The listing builds one solid part. Answer for the finished solid, in the listing's coordinates (mm). A direction names the side the tool comes from. Coordinates: 2 decimals unless noted, no trailing zeros. Write each loop counter-clockwise with the first axis right and the second up, starting at its lowest first coordinate (ties: lowest second). Pieces come first, ordered by that corner, then holes. Notation, with made-up numbers: M 28,7.5 L 32,7.5 A19 ccw 32,23.5 Z; hole C 88,-32.75 d6. An arc over 180 degrees is marked long. Answer as CSV lines item,"result".
```python
from build123d import *

# Parameters (mm, degrees)
F0_W     = 306.0534086764
F0_H     = 101.6
F0_W_2   = 101.6
F0_H_2   = 152.4
F0_W_3   = 100.3465913236
F1_DEPTH = 25.4


with BuildPart() as f1:
    # F0 (on Top) → F1 (new body)
    with BuildSketch(Plane.XY):
        with Locations((220.9462343127, 820.6196134418)):
            Rectangle(F0_W, F0_H)
        with Locations((220.9462343127, 566.6196134418)):
            Rectangle(F0_W, F0_H)
        with Locations((220.9462343127, 312.6196134418)):
            Rectangle(F0_W, F0_H)
        with Locations((220.9462343127, 58.6196134418)):
            Rectangle(F0_W, F0_H)
        with Locations((424.7729386508, 58.6196134418)):
            Rectangle(F0_W_2, F0_H)
        with Locations((424.7729386508, 185.6196134418)):
            Rectangle(F0_W_2, F0_H_2)
        with Locations((424.7729386508, 312.6196134418)):
            Rectangle(F0_W_2, F0_H)
        with Locations((424.7729386508, 439.6196134418)):
            Rectangle(F0_W_2, F0_H_2)
        with Locations((424.7729386508, 566.6196134418)):
            Rectangle(F0_W_2, F0_H)
        with Locations((424.7729386508, 693.6196134418)):
            Rectangle(F0_W_2, F0_H_2)
        with Locations((424.7729386508, 820.6196134418)):
            Rectangle(F0_W_2, F0_H)
        with Locations((17.7462343127, 820.6196134418)):
            Rectangle(F0_W_3, F0_H)
        with Locations((17.7462343127, 693.6196134418)):
            Rectangle(F0_W_3, F0_H_2)
        with Locations((17.7462343127, 566.6196134418)):
            Rectangle(F0_W_3, F0_H)
        with Locations((17.7462343127, 439.6196134418)):
            Rectangle(F0_W_3, F0_H_2)
        with Locations((17.7462343127, 312.6196134418)):
            Rectangle(F0_W_3, F0_H)
        with Locations((17.7462343127, 185.6196134418)):
            Rectangle(F0_W_3, F0_H_2)
        with Locations((17.7462343127, 58.6196134418)):
            Rectangle(F0_W_3, F0_H)
    extrude(amount=F1_DEPTH)


solid = f1.part
```
Q1. Find section C-C (x = 177). Give the vertices of the cut face in (y, z), and give its area (3 significant figures).
Output:
outline,"M 7.82,0 L 109.42,0 L 109.42,25.4 L 7.82,25.4 Z; M 261.82,0 L 363.42,0 L 363.42,25.4 L 261.82,25.4 Z; M 515.82,0 L 617.42,0 L 617.42,25.4 L 515.82,25.4 Z; M 769.82,0 L 871.42,0 L 871.42,25.4 L 769.82,25.4 Z"
area,"10,300 mm2"
Q2. Find section B-B (z = 8). Give the vertices of the cut face in (x, y).
Output:
outline,"M -32.43,7.82 L 475.57,7.82 L 475.57,871.42 L -32.43,871.42 Z; hole M 67.92,109.42 L 373.97,109.42 L 373.97,261.82 L 67.92,261.82 Z; hole M 67.92,363.42 L 373.97,363.42 L 373.97,515.82 L 67.92,515.82 Z; hole M 67.92,617.42 L 373.97,617.42 L 373.97,769.82 L 67.92,769.82 Z"
Q3. Find section A-A (y = 434.5). Give the vertices of the cut face in (x, z), and give its area (3 significant figures).
Output:
outline,"M -32.43,0 L 67.92,0 L 67.92,25.4 L -32.43,25.4 Z; M 373.97,0 L 475.57,0 L 475.57,25.4 L 373.97,25.4 Z"
area,"5,130 mm2"
Q4. The mould has two halves that part along X. Classify faces 1 (the flat face through (218, 542, 25.4)), 2 (the flat face through (223, 109.42, 13)), 3 (the flat face through (475.573, 434, 13)), 4 (the flat face through (-32.427, 446, 13)): pulls with the +X half, pulls with the -X half, needs draft (parallel to the pull), parting line crosses it, or undercut.
Output:
face 1,"needs draft"
face 2,"undercut"
face 3,"pulls with the +X half"
face 4,"pulls with the -X half"
Q5. For faces 5 (the flat face through (373.973, 439, 13)), 6 (the flat face through (218, 7.82, 13)), determine the directions among +Z, -Z, +X, -X, +Y, -Y from which every point of the face is accessible in a straight line to the end or side of a thin tool.
Output:
face 5,"+Z, -Z"
face 6,"+Z, -Z, +X, -X, -Y"
Q6. Straight lines are drawn through the part: line 1 (Y direction, x = 370, z = 20.5); line 2 (X direction, y = 505.5, z = 20). For each, find the intervals that lie inside material, in ascending order.
Output:
line 1,"7.82 to 109.42, 261.82 to 363.42, 515.82 to 617.42, 769.82 to 871.42"
line 2,"-32.43 to 67.92, 373.97 to 475.57"
